Verification items for the finished model (mm, model axes). Face numbers are marked on the shaded views. A direction names the side the tool comes from. Coordinates: 2 decimals unless noted, no trailing zeros. Loops run counter-clockwise (first coordinate to the right, second up) from the corner with the lowest first, then second, coordinate; pieces in that order, holes last. Notation, with made-up numbers: (-26.5, 16.5) -> (22.5, 16.5) arc R22 ccw to (22.5, 48.5) -> close; hole circle Ø1 at (-5, 80). An arc over 180 degrees is marked (long way). Write item = value, one per line.
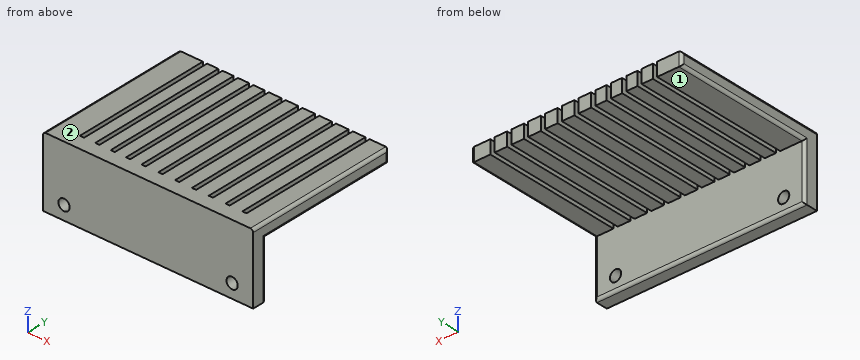
```python
from build123d import *

# Parameters (mm, degrees)
SKETCH1_W           = 150
SKETCH1_H           = 50
SKETCH1_R           = 4
BOSS_EXTRUDE1_DEPTH = 10
SKETCH2_W           = 150
SKETCH2_H           = 9.667678079
BOSS_EXTRUDE2_DEPTH = 100
SKETCH3_W           = 3
SKETCH3_H           = 100
CUT_EXTRUDE1_DEPTH  = 100
FILLET1_R           = 2


with BuildPart() as part:
    # Sketch1 → Boss-Extrude1 (new body)
    with BuildSketch(Plane(origin=(0, 0, 0), x_dir=(1, 0, 0), z_dir=(0, 1, 0))):
        Rectangle(SKETCH1_W, SKETCH1_H)
        with Locations((60, 15)):
            Circle(SKETCH1_R, mode=Mode.SUBTRACT)
        with Locations((-60, 15)):
            Circle(SKETCH1_R, mode=Mode.SUBTRACT)
    extrude(amount=BOSS_EXTRUDE1_DEPTH)

    # Sketch2 → Boss-Extrude2 (add)
    with BuildSketch(Plane(origin=(0, 10, 0), x_dir=(1, 0, 0), z_dir=(0, 1, 0))):
        with Locations((0, -20.166160961)):
            Rectangle(SKETCH2_W, SKETCH2_H)
    extrude(amount=BOSS_EXTRUDE2_DEPTH)

    # Sketch3 → Cut-Extrude1 (cut)
    with BuildSketch(Plane(origin=(0, 0, 15.332321921), x_dir=(-1, 0, 0), z_dir=(0, 0, -1))):
        with Locations((-12, 60)):
            Rectangle(SKETCH3_W, SKETCH3_H)
        with Locations((0, 60)):
            Rectangle(SKETCH3_W, SKETCH3_H)
        with Locations((12, 60)):
            Rectangle(SKETCH3_W, SKETCH3_H)
        with Locations((23, 60)):
            Rectangle(SKETCH3_W, SKETCH3_H)
        with Locations((34, 60)):
            Rectangle(SKETCH3_W, SKETCH3_H)
        with Locations((45, 60)):
            Rectangle(SKETCH3_W, SKETCH3_H)
        with Locations((56, 60)):
            Rectangle(SKETCH3_W, SKETCH3_H)
        with Locations((-24, 60)):
            Rectangle(SKETCH3_W, SKETCH3_H)
        with Locations((-36, 60)):
            Rectangle(SKETCH3_W, SKETCH3_H)
        with Locations((-48, 60)):
            Rectangle(SKETCH3_W, SKETCH3_H)
        with Locations((-60, 60)):
            Rectangle(SKETCH3_W, SKETCH3_H)
    extrude(amount=-CUT_EXTRUDE1_DEPTH, mode=Mode.SUBTRACT)

    # Fillet1
    fillet1_edges = [part.edges().sort_by_distance(p)[0] for p in [
        (0, 10, -25),
        (75, 10, -4.83383904),
        (-75, 60, 15.332321921),
        (75, 60, 15.332321921),
        (-75, 110, 20.16616096),
        (75, 110, 20.16616096),
        (-75, 10, -4.83383904),
        (75, 55, 25),
        (-75, 55, 25),
    ]]
    fillet(fillet1_edges, radius=FILLET1_R)


solid = part.part
```
1) Sectioned sample at D-D, the plane y = 79.5. Count the separate pieces of the cut face and the enclosed holes in it, plus the area to 3 significant figures.
Ans:
separate_pieces = 12
enclosed_holes = 0
area = 1,130 mm2
2) Depth check by flat-ended pin: pin 1 Ø2 at (y, z) = (13.5, 13.5) entering from +X; pin 2 Ø5 at (y, z) = (12, 8) entering from -X; pin 3 Ø6 at (y, z) = (84, 13) entering from -X; pin 4 Ø4.5 at (x, y) = (29.5, 57) entering from -Z. Enter the tip coordinate at first touch or a pass-through.
Ans:
pin_1 = through
pin_2 = -74.32
pin_3 = -74.49
pin_4 = 15.33
3) Sectioned sample at C-C, the plane z = 4.5. Record the cut outline in (x, y).
Ans:
outline = (-75, 0) -> (75, 0) -> (75, 8) arc R2 ccw to (73, 10) -> (-73, 10) arc R2 ccw to (-75, 8) -> close
4) Material ranges on line 1 (X direction, y = 4, z = -15); line 2 (Z direction, x = -60, y = 5.25); line 3 (X direction, y = 7.5, z = -11.5), recorded low to high.
Ans:
line_1 = -75 to -64, -56 to 56, 64 to 75
line_2 = -25 to -19, -11 to 25
line_3 = -75 to -61.94, -58.06 to 58.06, 61.94 to 75
5) Sectioned sample at B-B, the plane z = -15. Record the cut outline in (x, y).
Ans:
outline = (-75, 0) -> (-64, 0) -> (-64, 10) -> (-73, 10) arc R2 ccw to (-75, 8) -> close; (-56, 0) -> (56, 0) -> (56, 10) -> (-56, 10) -> close; (64, 0) -> (75, 0) -> (75, 8) arc R2 ccw to (73, 10) -> (64, 10) -> close
6) Sectioned sample at A-A, the plane x = -60. Record the cut outline in (y, z).
Ans:
outline = (0, -25) -> (8, -25) arc R2 ccw to (10, -23) -> (10, -19) -> (0, -19) -> close; (0, -11) -> (10, -11) -> (10, 15.33) -> (110, 15.33) -> (110, 25) -> (0, 25) -> close
7) Tool access check on the marked faces 1 and 2. Record the directions out of +Z, -Z, +X, -X, +Y, -Y that give a thin tool (end or side, any length) a straight path to the whole face; none if there is none.
Ans:
face_1 = -Z, +X, -X, +Y
face_2 = +Z, +X, -X, +Y, -Y
